Geometry check sheet. Reference: drawing and pictorial views, mm from the part's lowest x, y, z. Round coordinates to 2 decimals unless told otherwise and drop trailing zeros. Order: outer loops, then holes, each group sorted by start corner. A loop starts at its lowest first (then second) coordinate and runs counter-clockwise, first axis right, second up.
(1) Thickness scan on L1, parallel to X at y = 140.5, z = 120; L2, parallel to Y at x = 35, z = 27.5; L3, parallel to Z at x = 45, y = 38. Record the ranges inside material, lowest first.
(2) Cross-section at C-C on z = 120. Enter the section's corners in (x, y), and give its area (3 significant figures).
(3) Cross-section at B-B on y = 160. Enter the section's corners in (x, z), and give its area (3 significant figures).
(4) Draft check along Z on the marked faces 1, 2 and 3. Enter one of: pulls with the +Z half, pulls with the -Z half, needs draft (parallel to the pull), parting line crosses it, or undercut.
(5) Cross-section at D-D on y = 35. Enter the section's corners in (x, z).
(6) Gauge pin test, flat ends, axial feed: P1, Ø12, axis at x = 30, z = 40, coming from the +Y side; P2, Ø3, axis at y = 137.5, z = 121.5, coming from the -X side; P3, Ø4, axis at y = 28, z = 19.5, coming from the +X side; P4, Ø24, axis at x = 33, y = 117.5, coming from the -Z side. Record the tip position at first contact, or that the pin passes through.
(7) Cross-section at A-A on x = 35. Enter the section's corners in (y, z).
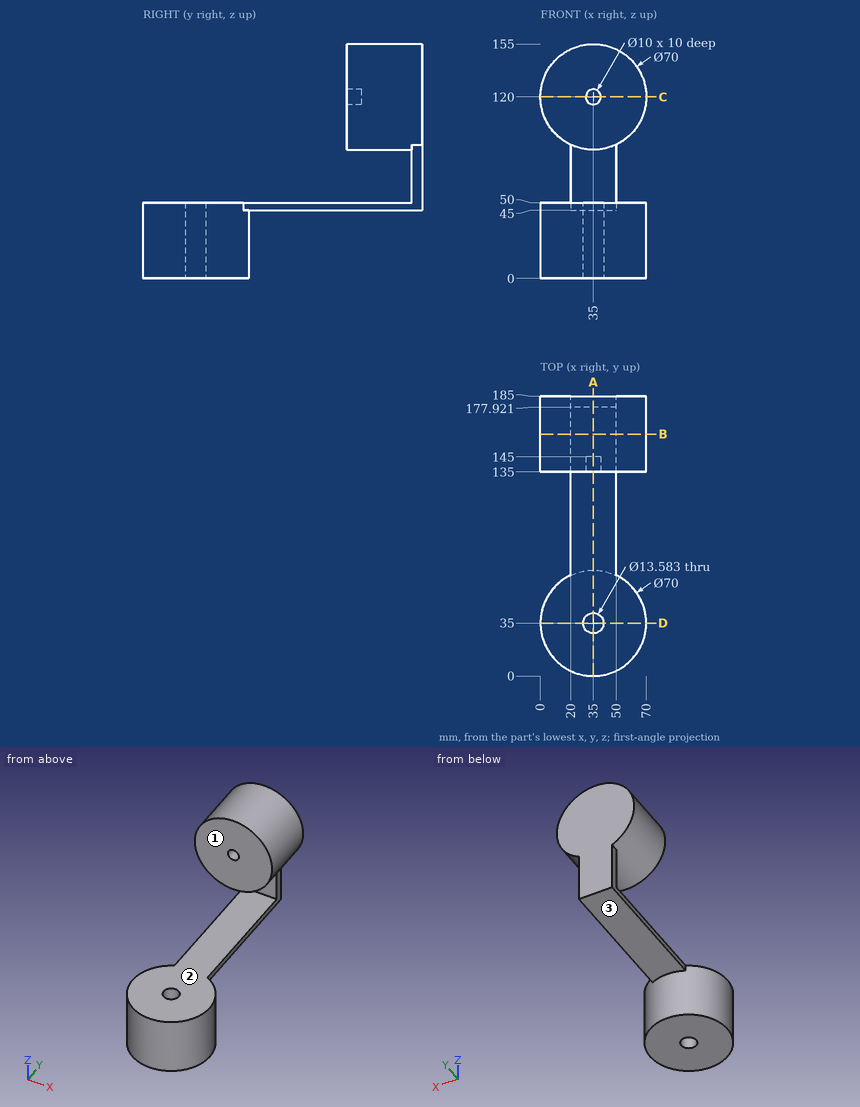
Found:
1. L1: x = 0 to 30, 40 to 70
1. L2: y = 0 to 28.21, 41.79 to 70
1. L3: z = 0 to 50
2. outline: (0, 135) - (30, 135) - (30, 145) - (40, 145) - (40, 135) - (70, 135) - (70, 185) - (0, 185) - close
2. area: 3,400 mm2
3. outline: circle Ø70 at (35, 120); (20, 45) - (50, 45) - (50, 50) - (20, 50) - close
3. area: 4,000 mm2
4. face 1: needs draft
4. face 2: undercut
4. face 3: pulls with the -Z half
5. outline: (0, 0) - (28.21, 0) - (28.21, 50) - (0, 50) - close; (41.79, 0) - (70, 0) - (70, 50) - (41.79, 50) - close
6. P1: stops at y = 185
6. P2: stops at x = 0
6. P3: stops at x = 69.64
6. P4: stops at z = 45
7. outline: (0, 0) - (28.21, 0) - (28.21, 50) - (0, 50) - close; (41.79, 0) - (70, 0) - (70, 45) - (185, 45) - (185, 155) - (135, 155) - (135, 125) - (145, 125) - (145, 115) - (135, 115) - (135, 85) - (177.92, 85) - (177.92, 50) - (41.79, 50) - close
